```python
from build123d import *

# Parameters (mm, degrees)
SKETCH1_R           = 1.65
BOSS_EXTRUDE1_DEPTH = 10
CUT_EXTRUDE1_DEPTH  = 29
CUT_EXTRUDE2_START  = -25
CUT_EXTRUDE2_DEPTH  = 30


with BuildPart() as part:
    # Sketch1 → Boss-Extrude1 (new body)
    with BuildSketch(Plane.XY):
        with BuildLine():
            Line((52.062696878, 9.140164993), (-10.937303122, 9.140164993))
            ThreePointArc((-10.937303122, 9.140164993), (-12.278943909, 8.823446566), (-13.337303122, 7.940164993))
            ThreePointArc((-13.337303122, 7.940164993), (-21.437303122, 10.640164993), (-13.337303122, 13.340164993))
            ThreePointArc((-13.337303122, 13.340164993), (-12.278943909, 12.45688342), (-10.937303122, 12.140164993))
            Line((-10.937303122, 12.140164993), (52.062696878, 12.140164993))
            ThreePointArc((52.062696878, 12.140164993), (52.769803659, 11.847271774), (53.062696878, 11.140164993))
            Line((53.062696878, 11.140164993), (53.062696878, 10.140164993))
            ThreePointArc((53.062696878, 10.140164993), (52.769803659, 9.433058211), (52.062696878, 9.140164993))
        make_face()
        with Locations((-16.937303122, 10.640164993)):
            Circle(SKETCH1_R, mode=Mode.SUBTRACT)
    extrude(amount=BOSS_EXTRUDE1_DEPTH)

    # Sketch7 → Cut-Extrude1 (cut)
    with BuildSketch(Plane(origin=(0, 0, 0), x_dir=(0, 0, -1), z_dir=(1, 0, 0))):
        Polygon((-8, 15.140164993), (-5, 12.140164993), (-2, 15.140164993), align=None)
    extrude(amount=-CUT_EXTRUDE1_DEPTH, mode=Mode.SUBTRACT)

    # Sketch8 → Cut-Extrude2 (cut)
    with BuildSketch(Plane(origin=(53.062696878, 0, 0), x_dir=(0, 0, -1), z_dir=(1, 0, 0)).offset(CUT_EXTRUDE2_START)):
        Polygon((0, 11.140164993), (-0.5, 10.640164993), (0, 10.140164993), align=None)
    cut_extrude2 = extrude(amount=-CUT_EXTRUDE2_DEPTH, mode=Mode.SUBTRACT)

    # Mirror1: Cut-Extrude2 across plane
    add(cut_extrude2.mirror(Plane(origin=(0, 0, 5), x_dir=(1, 0, 0), z_dir=(0, 0, -1))), mode=Mode.SUBTRACT)


solid = part.part
```
For this review, take the finished solid that the model builds, in its own axes (mm). A direction names the side the tool comes from. Give positions to 0.01 mm unless a question says otherwise; leave off trailing zeros. Order: outer loops, then holes, each group sorted by start corner. A loop starts at its lowest first (then second) coordinate and runs counter-clockwise, first axis right, second up.
1) Take a section at D-D (y = 7.25). Give the boundary of the cut face in (x, z).
2) Take a section at A-A (z = 8.75). Give the boundary of the cut face in (x, y), then the cut area to 3 significant figures.
3) Take a section at C-C (x = 29). Give the boundary of the cut face in (y, z), then the cut area to 3 significant figures.
4) The part is to be moulded in two halves that separate along X. For faces 6 (the face through (-20.68, 8.14, 4.93)), 7 (the face through (-17.29, 9.03, 4.93)), 8 (the face through (-17.12, 13.33, 6.19)), 9 (the face through (-12.296, 12.466, 7.465)), say which applies: released by +X, released by -X, zero draft, split by the parting line, or undercut.
5) Wall thickness on line 1 (X direction, y = 10.5, z = 1.25); line 2 (Y direction, x = 21.5, z = 5.25); line 3 (X direction, y = 11.75, z = 9): over which ranges is each line inside the solid? List them lowest first.
6) Take a section at B-B (x = 13.5). Give the boundary of the cut face in (y, z), then the cut area to 3 significant figures.
7) For faces 1 (the face through (20, 12.14, 5)), 2 (the face through (-17.12, 13.29, 3.85)), 3 (the face through (21, 9.14, 5)), 4 (the face through (10.5, 11.3, 10)), 5 (the face through (10.5, 11.3, 0)), list the 3-axis set-ups (+Z, -Z, +X, -X, +Y, -Y) from which the entire face can be reached by the end or side of a thin tool; tool diameter is ignored.
8) Insertion check: pin 1 (1 mm diameter, centred on x = 33.5, z = 9, fed in from -Y); pin 2 (3 mm diameter, centred on y = 8, z = 8, fed in from +X); pin 3 (1.5 mm diameter, centred on x = 20.5, y = 7, fed in from -Z); pin 4 (6 mm diameter, centred on x = -14, z = 3.5, fed in from +Y). Each pin has a flat end and moves straight along its axis. Give the tip position at first contact, or say it passes through.
Derived:
1. outline: (-19.9, 0) - (-13.98, 0) - (-13.98, 10) - (-19.9, 10) - close
2. outline: (-13.34, 7.94) arc R3 cw to (-10.94, 9.14) - (52.06, 9.14) arc R1 ccw to (53.06, 10.14) - (53.06, 11.14) arc R1 ccw to (52.06, 12.14) - (-10.94, 12.14) arc R3 cw to (-13.34, 13.34) arc R4.5 ccw (long way) to start; hole circle Ø3.3 at (-16.94, 10.64)
2. area: 252 mm2
3. outline: (9.14, 0) - (12.14, 0) - (12.14, 10) - (9.14, 10) - close
3. area: 30.0 mm2
4. face 6: split by the parting line
4. face 7: undercut
4. face 8: zero draft
4. face 9: released by +X
5. line 1: x = -21.44 to -18.58, -15.29 to 53.06
5. line 2: y = 9.14 to 12.14
5. line 3: x = -21.3 to -18.16, -15.72 to 52.86
6. outline: (9.14, 0) - (10.14, 0) - (10.64, 0.5) - (11.14, 0) - (12.14, 0) - (12.14, 10) - (11.14, 10) - (10.64, 9.5) - (10.14, 10) - (9.14, 10) - close
6. area: 29.5 mm2
7. face 1: +Z, -Z, +X, +Y
7. face 2: +X, -X, +Y
7. face 3: +Z, -Z, +X, -Y
7. face 4: +Z, +X, -X, +Y, -Y
7. face 5: -Z, +X, -X, +Y, -Y
8. pin 1: stops at y = 9.14
8. pin 2: stops at x = 52.83
8. pin 3: passes through
8. pin 4: stops at y = 15.13
